For this review, take the finished solid that the model builds, in its own axes (mm). A direction names the side the tool comes from. Coordinates: 2 decimals unless noted, no trailing zeros. Write each loop counter-clockwise with the first axis right and the second up, starting at its lowest first coordinate (ties: lowest second). Pieces come first, ordered by that corner, then holes. Notation, with made-up numbers: (-37.5, -19.5) - (9.5, -19.5) arc R13 ccw to (9.5, 5.5) - close; hole circle Ø6 at (49, 86.5). An arc over 180 degrees is marked (long way). Use one line per item in the form item = value. Start each with the question number.
1) We need section C-C (z = 2). Give the boundary of the cut face in (x, y), plus the area to 3 significant figures.
2) Insertion check: P1, Ø2.5, axis at x = 0.5, z = -3.5, coming from the +Y side; P2, Ø4, axis at y = 52, z = -2.5, coming from the +X side; P3, Ø3.5, axis at y = 31.5, z = -4, coming from the +X side. Each pin has a flat end and moves straight along its axis. Give the tip position at first contact, or say it passes through.
3) Mouldability with a two-part tool opening along Z and no side actions: class faces 1 (the flat face through (0, 0, 0)), 2 (the flat face through (0, 45, 0)), 3 (the flat face through (0, 30, 0)), 4 (the cylindrical face through (-1.63, 29.58, 7.32)) as pulls with the +Z half, pulls with the -Z half, needs draft (parallel to the pull), parting line crosses it, or undercut.
4) We need section D-D (y = 21). Give the boundary of the cut face in (x, z) (3 decimals), plus the area to 3 significant figures.
5) For L1, parallel to X at y = 50.25, z = 0; L2, parallel to Y at x = -0.5, z = -1.5 (3 decimals), list the stretches that pass through material, from the lowest coordinate up. Write a range as from..to.
6) We need section B-B (x = 0). Give the boundary of the cut face in (y, z) (3 decimals).
7) We need section A-A (z = -1.75). Give the boundary of the cut face in (x, y) (3 decimals), plus the area to 3 significant figures.
8) Tool access review of faces 5 (the flat face through (2, 60, 5)), 6 (the flat face through (0, 19.875, -4)), 7 (the cylindrical face through (-1.08, 52.6, 4.88)): name each direction out of +Z, -Z, +X, -X, +Y, -Y from which nothing blocks a thin tool from reaching the whole face with its end or side.
```python
from build123d import *

# Parameters (mm, degrees)
SKETCH1_R           = 7.5
BOSS_EXTRUDE1_DEPTH = 60
SKETCH2_R           = 5
CUT_EXTRUDE1_DEPTH  = 15
SKETCH3_W           = 5.25
SKETCH3_H           = 20.25
CUT_EXTRUDE2_DEPTH  = 7.5


with BuildPart() as part:
    # Sketch1 → Boss-Extrude1 (new body)
    with BuildSketch(Plane(origin=(0, 0, 0), x_dir=(1, 0, 0), z_dir=(0, 1, 0))):
        Circle(SKETCH1_R)
    extrude(amount=BOSS_EXTRUDE1_DEPTH)

    # Sketch2 → Cut-Extrude1 (cut)
    with BuildSketch(Plane(origin=(0, 60, 0), x_dir=(1, 0, 0), z_dir=(0, 1, 0))):
        Circle(SKETCH2_R)
    extrude(amount=-CUT_EXTRUDE1_DEPTH, mode=Mode.SUBTRACT)

    # Sketch3 → Cut-Extrude2 (cut)
    with BuildSketch(Plane(origin=(0, 0, -7.5), x_dir=(-1, 0, 0), z_dir=(0, 0, -1))):
        with Locations((0, 30)):
            Rectangle(SKETCH3_W, SKETCH3_H)
    extrude(amount=-CUT_EXTRUDE2_DEPTH, mode=Mode.SUBTRACT)


solid = part.part
```
Determined:
q1.outline = (-7.23, 0) - (7.23, 0) - (7.23, 60) - (4.58, 60) - (4.58, 45) - (-4.58, 45) - (-4.58, 60) - (-7.23, 60) - close
q1.area = 730 mm²
q2.P1 = 45
q2.P2 = 7.48
q2.P3 = 7.15
q3.face_1 = needs draft
q3.face_2 = undercut
q3.face_3 = pulls with the -Z half
q3.face_4 = parting line crosses it
q4.outline = (-2.625, -7.026) - (-2.625, 0) - (2.625, 0) - (2.625, -7.026) arc R7.5 ccw (long way) to start
q4.area = 138 mm²
q5.L1 = -7.5..-5, 5..7.5
q5.L2 = 0..19.875, 40.125..45
q6.outline = (0, -7.5) - (19.875, -7.5) - (19.875, 0) - (40.125, 0) - (40.125, -7.5) - (60, -7.5) - (60, -5) - (45, -5) - (45, 5) - (60, 5) - (60, 7.5) - (0, 7.5) - close
q7.outline = (-7.293, 0) - (7.293, 0) - (7.293, 60) - (4.684, 60) - (4.684, 45) - (-4.684, 45) - (-4.684, 60) - (-7.293, 60) - close; hole (-2.625, 19.875) - (2.625, 19.875) - (2.625, 40.125) - (-2.625, 40.125) - close
q7.area = 628 mm²
q8.face_5 = +Z, -Z, +X, -X, +Y
q8.face_6 = -Z
q8.face_7 = +Y
